Read the model definition and answer for the solid it produces. Units are mm, in the model's axes. A direction names the side the tool comes from. Give positions to 0.01 mm unless a question says otherwise; leave off trailing zeros. Write each loop counter-clockwise with the first axis right and the second up, starting at its lowest first coordinate (ties: lowest second). Pieces come first, ordered by that corner, then holes. Notation, with made-up numbers: (26.25, 36.25) -> (76.25, 36.25) arc R10 cw to (76.25, 47.25) -> close; hole circle Ø3 at (-33, 55.5). An arc over 180 degrees is marked (long way). Use a Markdown table: item, result.
from build123d import *

# Parameters (mm, degrees)
SKETCH016_R       = 1.85
EXTRUDE013_DEPTH  = 12
CYLINDER007_R     = 5
CYLINDER007_DEPTH = 1
EXTRUDE012_DEPTH  = 15


with BuildPart() as extrude013:
    # Sketch016 → Extrude013 (new body)
    with BuildSketch(Plane.XZ):
        Polygon((11.75, 36), (11.75, 19), (-17.25, 19), (-23.25, 25), (-23.25, 30), (-17.25, 36), align=None)
        with Locations((-16, 27.481564)):
            Circle(SKETCH016_R, mode=Mode.SUBTRACT)
    extrude(amount=-EXTRUDE013_DEPTH)


with BuildPart() as unprintable:
    # Cylinder007 → Cylinder007 (new body)
    with BuildSketch(Plane(origin=(-16, 18, 27.5), x_dir=(1, 0, 0), z_dir=(0, -1, 0))):
        Circle(CYLINDER007_R)
    extrude(amount=CYLINDER007_DEPTH)


with BuildPart() as body007:
    # Sketch015 → Extrude012 (new body)
    with BuildSketch(Plane.XY.offset(50)):
        with BuildLine():
            ThreePointArc((8.75, 0), (1.006685, 8.691898), (-8.518363, 2))
            Line((-8.518363, 2), (-22.518363, 2))
            Line((-22.518363, 4), (-22.518363, 2))
            Line((-9.978101, 4), (-22.518363, 4))
            ThreePointArc((10.75, 0), (2.036899, 10.555261), (-9.978101, 4))
            Line((8.75, 0), (10.75, 0))
        make_face()
    extrude(amount=EXTRUDE012_DEPTH)


with BuildPart() as body007_1:
    # Extrude012 placement: moved
    add(body007.part.moved(Location((0, 0, -30))))

    # Fusion016: union unprintable
    add(unprintable.part)

    # Common001: intersect Extrude013
    add(extrude013.part, mode=Mode.INTERSECT)


with BuildPart() as part_mirroring008:
    # Part__Mirroring008: instance of Body007
    add(body007_1.part.mirror(Plane(origin=(0, 0, 0), x_dir=(1, 0, 0), z_dir=(0, 1, 0))))


solid = part_mirroring008.part
Item 1: A cutting plane is placed at C-C (z = 21). Give the vertices of the cut face in (x, y), then the cut area to 3 significant figures.
Return value:
| item | result |
|---|---|
| outline | (-19.25, -4) -> (-9.98, -4) arc R10.75 ccw to (10.75, 0) -> (8.75, 0) arc R8.75 cw to (-8.52, -2) -> (-19.25, -2) -> close |
| area | 75.1 mm^2 |
Item 2: A tool of negligible diameter and unlimited length cuts with its end or side. For faces 5 (the face through (-20.35, -2.99, 22.1)), 6 (the face through (-14.8, -4, 25.7)), from which of +Z, -Z, +X, -X, +Y, -Y can it reach the whole face along a straight path? Write none if from no direction.
Return value:
| item | result |
|---|---|
| face 5 | -Z, -X, +Y, -Y |
| face 6 | +Z, -Z, -X, -Y |
Item 3: A cutting plane is placed at A-A (x = -16). Give the vertices of the cut face in (y, z).
Return value:
| item | result |
|---|---|
| outline | (-4, 20) -> (-2, 20) -> (-2, 25.63) -> (-4, 25.63) -> close; (-4, 29.33) -> (-2, 29.33) -> (-2, 35) -> (-4, 35) -> close |
Item 4: A cutting plane is placed at D-D (z = 29). Give the vertices of the cut face in (x, y).
Return value:
| item | result |
|---|---|
| outline | (-22.52, -4) -> (-17.06, -4) -> (-17.06, -2) -> (-22.52, -2) -> close; (-14.94, -4) -> (-9.98, -4) arc R10.75 ccw to (10.75, 0) -> (8.75, 0) arc R8.75 cw to (-8.52, -2) -> (-14.94, -2) -> close |
Item 5: Straight lines are drawn through the part: line 1 along Z through (x, y) = (-16, -2.7); line 2 along Y through (x, z) = (-20.5, 23.75); line 3 along X through (y, z) = (-3, 29.5). For each, find the intervals that lie inside material, in ascending order. Write a range as [from, to].
Return value:
| item | result |
|---|---|
| line 1 | [20, 25.63], [29.33, 35] |
| line 2 | [-4, -2] |
| line 3 | [-22.52, -8.22], [8.22, 10.32] |
Item 6: A cutting plane is placed at B-B (y = -7.75). Give the vertices of the cut face in (x, z), then the cut area to 3 significant figures.
Return value:
| item | result |
|---|---|
| outline | (-7.45, 20) -> (-4.06, 20) -> (-4.06, 35) -> (-7.45, 35) -> close; (4.06, 20) -> (7.45, 20) -> (7.45, 35) -> (4.06, 35) -> close |
| area | 102 mm^2 |
Item 7: Each of these flat-tipped pins is pushed along its axis until it touches: P1, Ø6, axis at x = -11, z = 32.5, coming from the -Y side; P2, Ø6.5, axis at x = -18, z = 28, coming from the -Y side; P3, Ø4, axis at x = -11, y = -8, coming from the +Z side; P4, Ø4, axis at x = -19, z = 24.5, coming from the +Y side. Where does it stop, or does it pass through?
Return value:
| item | result |
|---|---|
| P1 | y = -7.18 |
| P2 | y = -4 |
| P3 | through |
| P4 | y = -2 |
Item 8: For a pull along X with two mould halves and no side action, classify faces 1 (the face through (2.24, -10.514, 27.395)), 2 (the face through (-15.15, -2.99, 25.84)), 3 (the face through (-20.41, -2.99, 32.84)), 4 (the face through (-14, -2, 27)) as +X half, -X half, draft (parallel to the pull), parting line (faces both ways), or undercut.
Return value:
| item | result |
|---|---|
| face 1 | parting line |
| face 2 | undercut |
| face 3 | -X half |
| face 4 | draft |
